CAD build for the part. Positions are in the model's coordinates, mm. A direction names the side the tool comes from. Round coordinates to 2 decimals unless told otherwise and drop trailing zeros. Write each loop counter-clockwise with the first axis right and the second up, starting at its lowest first coordinate (ties: lowest second). Pieces come first, ordered by that corner, then holes. Notation, with made-up numbers: (54, 2.25) - (98, 2.25) arc R28 ccw to (98, 36.25) - close; hole circle Ø6 at (17, -18). An arc over 180 degrees is marked (long way). Use one line per item in the form item = value. Start each with the question number.
Item 1: Band-saw the part on B-B, the plane z = 7. Give the number of separate pieces and of enclosed holes in the cut face, and give its area (3 significant figures).
Item 2: Band-saw the part on C-C, the plane y = -11.5. List the corners of the cut face in (x, z), and give its area (3 significant figures).
Item 3: Tool access for faces 4 (the flat face through (20.45, -10, 2)), 5 (the flat face through (-17.55, 0, 4)), 6 (the flat face through (-20.45, 10, 2)), 7 (the flat face through (0, -17.1, 6)): list every direction of +Z, -Z, +X, -X, +Y, -Y with a clear straight run to the whole face (end or side of a thin tool).
Item 4: Pin check, flat tips, straight feed: pin 1 (2.5 mm diameter, centred on y = 3.5, z = 2, fed in from -X); pin 2 (4 mm diameter, centred on x = 9.5, y = -11.5, fed in from +Z). Stop position of each tip, or through.
Item 5: Drill centre lines: L1, parallel to Y at x = 13, z = 6.5; L2, parallel to Y at x = 18, z = 6.5; L3, parallel to Y at x = -21, z = 0.5. Where is each one in solid material? Low to high.
Item 6: Pull direction Y, two halves, no side cores. Call faces 1 (the flat face through (20.45, 10, 2)), 2 (the flat face through (0, -18.9, 4)), 3 (the flat face through (0, -18, 8)): +Y half, -Y half, draft (parallel to the pull), parting line (faces both ways), or undercut.
Item 7: Band-saw the part on A-A, the plane x = -16.5. List the corners of the cut face in (y, z), and give its area (3 significant figures).
Item 8: Band-saw the part on D-D, the plane y = -4. List the corners of the cut face in (x, z).
from build123d import *

# Parameters (mm, degrees)
F0_W      = 53.5
F0_H      = 37.8
F1_DEPTH  = 8
F2_W      = 53.5
F2_H      = 8
F3_DEPTH  = 3.25
F4_W      = 9.9
F4_H      = 8
F5_DEPTH  = 9.2
F5_TAPER  = -12
F6_W      = 9.9
F6_H      = 8
F7_DEPTH  = 9.2
F7_TAPER  = -12
F9_W      = 6.3
F9_H      = 1.2
F8_W      = 6.3
F8_H      = 1.2
F10_DEPTH = 4.75


with BuildPart() as f1:
    # F0 (on Top) → F1 (new body)
    with BuildSketch(Plane.XY):
        Rectangle(F0_W, F0_H)
    extrude(amount=F1_DEPTH)

    # F2 (on face) → F3 (cut)
    with BuildSketch(Plane.XY.offset(8)):
        with Locations((0, -13.1)):
            Rectangle(F2_W, F2_H)
        with Locations((0, 13.1)):
            Rectangle(F2_W, F2_H)
    extrude(amount=-F3_DEPTH, mode=Mode.SUBTRACT)

    # F4 (on face) → F5 (cut)
    with BuildSketch(Plane(origin=(-26.75, 0, 0), x_dir=(0, -1, 0), z_dir=(-1, 0, 0))):
        with Locations((0, 4)):
            Rectangle(F4_W, F4_H)
    extrude(amount=-F5_DEPTH, taper=F5_TAPER, mode=Mode.SUBTRACT)

    # F6 (on face) → F7 (cut)
    with BuildSketch(Plane.YZ.offset(26.75)):
        with Locations((0, 4)):
            Rectangle(F6_W, F6_H)
    extrude(amount=-F7_DEPTH, taper=F7_TAPER, mode=Mode.SUBTRACT)

    # F9 (on face) + F8 (on face) → F10 (cut)
    with BuildSketch(Plane.XY.offset(4.75)):
        with Locations((23.6, 9.7)):
            Rectangle(F9_W, F9_H)
        with Locations((-23.6, 9.7)):
            Rectangle(F9_W, F9_H)
    with BuildSketch(Plane.XY.offset(4.75)):
        with Locations((-23.6, -9.7)):
            Rectangle(F8_W, F8_H)
        with Locations((23.6, -9.7)):
            Rectangle(F8_W, F8_H)
    extrude(amount=-F10_DEPTH, mode=Mode.SUBTRACT)


solid = f1.part
Determined:
q1.separate_pieces = 3
q1.enclosed_holes = 0
q1.area = 948 mm²
q2.outline = (-26.75, 0) - (26.75, 0) - (26.75, 4.75) - (-26.75, 4.75) - close
q2.area = 254 mm²
q3.face_4 = +Z, -Z, +X
q3.face_5 = +Z, -Z
q3.face_6 = +Z, -Z, -X
q3.face_7 = +Z, +X, -X
q4.pin_1 = -17.55
q4.pin_2 = 4.75
q5.L1 = -18.9 to -17.1, -9.1 to 9.1, 17.1 to 18.9
q5.L2 = -18.9 to -17.1, -9.1 to -6.81, 6.81 to 9.1, 17.1 to 18.9
q5.L3 = -18.9 to -10.3, -9.1 to -6.17, 6.17 to 9.1, 10.3 to 18.9
q6.face_1 = undercut
q6.face_2 = -Y half
q6.face_3 = draft
q7.outline = (-18.9, 0) - (18.9, 0) - (18.9, 8) - (17.1, 8) - (17.1, 4.75) - (9.1, 4.75) - (9.1, 8) - (-9.1, 8) - (-9.1, 4.75) - (-17.1, 4.75) - (-17.1, 8) - (-18.9, 8) - close
q7.area = 250 mm²
q8.outline = (-17.55, 0) - (17.55, 0) - (17.55, 8) - (-17.55, 8) - close
